Design review of the part built by this model. Coordinates are the model's own, in mm. A direction names the side the tool comes from. Coordinates: 2 decimals unless noted, no trailing zeros. Loops run counter-clockwise (first coordinate to the right, second up) from the corner with the lowest first, then second, coordinate; pieces in that order, holes last. Notation, with made-up numbers: (-15.75, 23.5) - (21.25, 23.5) arc R17 cw to (21.25, 43.5) - close; hole circle Ø4 at (-39, -20). An arc over 180 degrees is marked (long way). Return JSON: item names as keys, results as strings. Group by question number.
from build123d import *

# Parameters (mm, degrees)
BOSS_EXTRUDE1_DEPTH = 150
SKETCH2_R           = 4.25
CUT_EXTRUDE1_DEPTH  = 21


with BuildPart() as part:
    # Sketch1 → Boss-Extrude1 (new body)
    with BuildSketch(Plane.XY):
        with BuildLine():
            Line((-9, 10), (9, 10))
            ThreePointArc((9, 10), (9.707106781, 9.707106781), (10, 9))
            Line((10, 9), (10, -9))
            ThreePointArc((10, -9), (9.707106781, -9.707106781), (9, -10))
            Line((9, -10), (-9, -10))
            ThreePointArc((-9, -10), (-9.707106781, -9.707106781), (-10, -9))
            Line((-10, -9), (-10, 9))
            ThreePointArc((-10, 9), (-9.707106781, 9.707106781), (-9, 10))
        make_face()
        with BuildLine():
            Line((-7, 8), (7, 8))
            ThreePointArc((7, 8), (7.707106781, 7.707106781), (8, 7))
            Line((8, 7), (8, -7))
            ThreePointArc((8, -7), (7.707106781, -7.707106781), (7, -8))
            Line((7, -8), (-7, -8))
            ThreePointArc((-7, -8), (-7.707106781, -7.707106781), (-8, -7))
            Line((-8, -7), (-8, 7))
            ThreePointArc((-8, 7), (-7.707106781, 7.707106781), (-7, 8))
        make_face(mode=Mode.SUBTRACT)
    extrude(amount=BOSS_EXTRUDE1_DEPTH)

    # Sketch2 → Cut-Extrude1 (cut, through all)
    with BuildSketch(Plane(origin=(10, 0, 0), x_dir=(0, 0, -1), z_dir=(1, 0, 0))):
        with Locations((-8, 0)):
            Circle(SKETCH2_R)
    extrude(amount=-CUT_EXTRUDE1_DEPTH, mode=Mode.SUBTRACT)


solid = part.part
Item 1: Add section D-D (z = 71.5). State the section outline as (x, y) points.
Item 2: To check wall thickness, follow line 1 (Y direction, x = 0.5, z = 95); line 2 (Y direction, x = 8.95, z = 8). State the ranges of each line that lie inside material, in increasing order. Write a range as from..to.
Item 3: Add section C-C (y = 0). State the section outline as (x, z) points, then the cut area to 3 significant figures.
Item 4: Add section A-A (z = 8). State the section outline as (x, y) points, then the cut area to 3 significant figures.
Item 5: Add section B-B (x = 1.25). State the section outline as (y, z) points, then the cut area to 3 significant figures.
Item 6: Draft analysis for pull direction X (two halves, no side actions). For faces 3 (the face through (8, 0, 74)), 4 (the face through (9, 0, 0)), 5 (the face through (10, 0, 74)), state which applies: pulls with the +X half, pulls with the -X half, needs draft (parallel to the pull), parting line crosses it, or undercut.
Item 7: For faces 1 (the face through (9, 0, 150)), 2 (the face through (0, 8, 74)), list the 3-axis set-ups (+Z, -Z, +X, -X, +Y, -Y) from which the entire face can be reached by the end or side of a thin tool; tool diameter is ignored.
Answers below:
{
 "1": {"outline": "(-10, -9) arc R1 ccw to (-9, -10) - (9, -10) arc R1 ccw to (10, -9) - (10, 9) arc R1 ccw to (9, 10) - (-9, 10) arc R1 ccw to (-10, 9) - close; hole (-8, -7) arc R1 ccw to (-7, -8) - (7, -8) arc R1 ccw to (8, -7) - (8, 7) arc R1 ccw to (7, 8) - (-7, 8) arc R1 ccw to (-8, 7) - close"},
 "2": {"line 1": "y = -10..-8, 8..10", "line 2": "y = -10..-4.25, 4.25..10"},
 "3": {"outline": "(-10, 0) - (-8, 0) - (-8, 3.75) - (-10, 3.75) - close; (-10, 12.25) - (-8, 12.25) - (-8, 150) - (-10, 150) - close; (8, 0) - (10, 0) - (10, 3.75) - (8, 3.75) - close; (8, 12.25) - (10, 12.25) - (10, 150) - (8, 150) - close", "area": "566 mm^2"},
 "4": {"outline": "(-10, -9) arc R1 ccw to (-9, -10) - (9, -10) arc R1 ccw to (10, -9) - (10, -4.25) - (8, -4.25) - (8, -7) arc R1 cw to (7, -8) - (-7, -8) arc R1 cw to (-8, -7) - (-8, -4.25) - (-10, -4.25) - close; (-10, 4.25) - (-8, 4.25) - (-8, 7) arc R1 cw to (-7, 8) - (7, 8) arc R1 cw to (8, 7) - (8, 4.25) - (10, 4.25) - (10, 9) arc R1 ccw to (9, 10) - (-9, 10) arc R1 ccw to (-10, 9) - close", "area": "110 mm^2"},
 "5": {"outline": "(-10, 0) - (-8, 0) - (-8, 150) - (-10, 150) - close; (8, 0) - (10, 0) - (10, 150) - (8, 150) - close", "area": "600 mm^2"},
 "6": {"face 3": "undercut", "face 4": "needs draft", "face 5": "pulls with the +X half"},
 "7": {"face 1": "+Z, +X, -X, +Y, -Y", "face 2": "+Z, -Z"}
}
